Read the model definition and answer for the solid it produces. Units are mm, in the model's axes. A direction names the side the tool comes from. Coordinates: 2 decimals unless noted, no trailing zeros. Order: outer loops, then holes, each group sorted by start corner. A loop starts at its lowest first (then second) coordinate and runs counter-clockwise, first axis right, second up.
```python
from build123d import *

# Parameters (mm, degrees)
SKETCH1_W           = 37.5
SKETCH1_H           = 37.5
BOSS_EXTRUDE1_DEPTH = 15
SHELL1_T            = 2.25
CUT_EXTRUDE1_REACH  = 52.026
SKETCH2_W           = 25
SKETCH2_H           = 11
CUT_EXTRUDE2_REACH  = 52.026
SKETCH3_W           = 18
SKETCH3_H           = 9
CUT_EXTRUDE3_REACH  = 36.345
SKETCH5_W           = 29
SKETCH5_H           = 29
FILLET1_R           = 2
CUT_EXTRUDE4_REACH  = 52.026
SKETCH6_W           = 22
SKETCH6_H           = 14
FILLET2_R           = 1
SKETCH9_W           = 12
SKETCH9_H           = 10
BOSS_EXTRUDE3_DEPTH = 5
BOSS_EXTRUDE4_DEPTH = 10
SKETCH11_R          = 1.65
CUT_EXTRUDE5_DEPTH  = 5
CUT_EXTRUDE6_REACH  = 42.989
SKETCH12_R          = 3
CUT_EXTRUDE7_REACH  = 44.75
MIRROR3_OUTLINE_R   = 1.65
MIRROR3_DEPTH       = 5
MIRROR3_START       = 5
MIRROR3_2_OUTLINE_R = 3
MIRROR3_2_DEPTH     = 12.25
MIRROR3_START_2     = 27.072732359
MIRROR3_3_OUTLINE_W = 20
MIRROR3_3_OUTLINE_H = 11
MIRROR3_3_DEPTH     = 9.927267641
CHAMFER1_SIZE       = 2
FILLET3_R           = 1


with BuildPart() as part:
    # Sketch1 → Boss-Extrude1 (new body)
    with BuildSketch(Plane(origin=(0, 0, 0), x_dir=(1, 0, 0), z_dir=(0, 1, 0))):
        Rectangle(SKETCH1_W, SKETCH1_H)
    extrude(amount=BOSS_EXTRUDE1_DEPTH)

    # Shell1
    shell1_openings = [part.faces().sort_by_distance(p)[0] for p in [
        (0, 0, 0),
    ]]
    offset(amount=SHELL1_T, openings=shell1_openings, kind=Kind.INTERSECTION)

    # Sketch2 → Cut-Extrude1 (cut, up to next)
    with BuildSketch(Plane.XY.offset(21), mode=Mode.PRIVATE) as cut_extrude1_sk1:
        with Locations((0, 5.5)):
            Rectangle(SKETCH2_W, SKETCH2_H)
    cut_extrude1_tool1 = extrude(cut_extrude1_sk1.sketch, amount=-CUT_EXTRUDE1_REACH, mode=Mode.PRIVATE) & part.part
    add(cut_extrude1_tool1.solids().sort_by_distance((0, 5.5, 21))[0], mode=Mode.SUBTRACT)

    # Sketch3 → Cut-Extrude2 (cut, up to next)
    with BuildSketch(Plane(origin=(21, 0, 0), x_dir=(0, 0, -1), z_dir=(1, 0, 0)), mode=Mode.PRIVATE) as cut_extrude2_sk1:
        with Locations((-2, 4.5)):
            Rectangle(SKETCH3_W, SKETCH3_H)
    cut_extrude2_tool1 = extrude(cut_extrude2_sk1.sketch, amount=-CUT_EXTRUDE2_REACH, mode=Mode.PRIVATE) & part.part
    add(cut_extrude2_tool1.solids().sort_by_distance((21, 4.5, 2))[0], mode=Mode.SUBTRACT)

    # Sketch5 → Cut-Extrude3 (cut, up to next)
    with BuildSketch(Plane(origin=(0, 17.25, 0), x_dir=(1, 0, 0), z_dir=(0, 1, 0)), mode=Mode.PRIVATE) as cut_extrude3_sk1:
        Rectangle(SKETCH5_W, SKETCH5_H)
    cut_extrude3_tool1 = extrude(cut_extrude3_sk1.sketch, amount=-CUT_EXTRUDE3_REACH, mode=Mode.PRIVATE) & part.part
    add(cut_extrude3_tool1.solids().sort_by_distance((0, 17.25, 0))[0], mode=Mode.SUBTRACT)

    # Fillet1
    fillet1_edges = [part.edges().sort_by_distance(p)[0] for p in [
        (14.5, 16.125, -14.5),
        (14.5, 16.125, 14.5),
        (-14.5, 16.125, 14.5),
        (-14.5, 16.125, -14.5),
    ]]
    fillet(fillet1_edges, radius=FILLET1_R)

    # Sketch6 → Cut-Extrude4 (cut, up to next)
    with BuildSketch(Plane(origin=(0, 0, -21), x_dir=(-1, 0, 0), z_dir=(0, 0, -1)), mode=Mode.PRIVATE) as cut_extrude4_sk1:
        with Locations((0, 7)):
            Rectangle(SKETCH6_W, SKETCH6_H)
    cut_extrude4_tool1 = extrude(cut_extrude4_sk1.sketch, amount=-CUT_EXTRUDE4_REACH, mode=Mode.PRIVATE) & part.part
    add(cut_extrude4_tool1.solids().sort_by_distance((0, 7, -21))[0], mode=Mode.SUBTRACT)

    # Fillet2
    fillet2_edges = [part.edges().sort_by_distance(p)[0] for p in [
        (-11, 14, -19.875),
        (11, 14, -19.875),
        (12.5, 11, 19.875),
        (-12.5, 11, 19.875),
        (19.875, 9, 11),
        (19.875, 9, -7),
    ]]
    fillet(fillet2_edges, radius=FILLET2_R)

    # Sketch9 → Boss-Extrude3 (add)
    with BuildSketch(Plane.XZ):
        with Locations((-27, 16)):
            Rectangle(SKETCH9_W, SKETCH9_H)
    boss_extrude3 = extrude(amount=-BOSS_EXTRUDE3_DEPTH)

    # Sketch10 → Boss-Extrude4 (add)
    with BuildSketch(Plane.XY.offset(21)):
        Polygon((-21, 17.25), (-33, 5), (-21, 5), align=None)
    boss_extrude4 = extrude(amount=-BOSS_EXTRUDE4_DEPTH)

    # Sketch11 → Cut-Extrude5 (cut)
    with BuildSketch(Plane.XZ):
        with Locations(Location((-28, 16, 0), (0, 0, 270))):
            Circle(SKETCH11_R)
    cut_extrude5 = extrude(amount=-CUT_EXTRUDE5_DEPTH, mode=Mode.SUBTRACT)

    # Cut-Extrude6: up to this plane
    cut_extrude6_end = Plane(origin=(-21, 17.25, -6.14825064), z_dir=(-0.7143585813751187, 0.6997798348164429, 0))
    # Sketch12 → Cut-Extrude6 (cut, up to the surface)
    with BuildSketch(Plane.XZ.offset(-5), mode=Mode.PRIVATE) as cut_extrude6_sk1:
        with Locations(Location((-28, 16, 0), (0, 0, 270))):
            Circle(SKETCH12_R)
    cut_extrude6_tool1 = split(extrude(cut_extrude6_sk1.sketch, amount=-CUT_EXTRUDE6_REACH, mode=Mode.PRIVATE), bisect_by=cut_extrude6_end, keep=Keep.BOTH, mode=Mode.PRIVATE)
    cut_extrude6 = cut_extrude6_tool1.solids().sort_by_distance((-28, 5, 16))[0]
    add(cut_extrude6, mode=Mode.SUBTRACT)

    # Cut-Extrude7: up to this plane
    cut_extrude7_end = Plane(origin=(-21, 17.25, -6.14825064), z_dir=(-0.7143585813751187, 0.6997798348164429, 0))
    # Sketch13 → Cut-Extrude7 (cut, up to the surface)
    with BuildSketch(Plane.XZ, mode=Mode.PRIVATE) as cut_extrude7_sk1:
        with BuildLine():
            ThreePointArc((-33, 16), (-31.535533906, 19.535533906), (-28, 21))
            Line((-28, 21), (-33, 21))
            Line((-33, 21), (-33, 16))
        make_face()
    cut_extrude7_tool1 = split(extrude(cut_extrude7_sk1.sketch, amount=-CUT_EXTRUDE7_REACH, mode=Mode.PRIVATE), bisect_by=cut_extrude7_end, keep=Keep.BOTH, mode=Mode.PRIVATE)
    # Sketch13 → Cut-Extrude7 (cut, up to the surface)
    with BuildSketch(Plane.XZ, mode=Mode.PRIVATE) as cut_extrude7_sk2:
        with BuildLine():
            Line((-33, 11), (-28, 11))
            ThreePointArc((-28, 11), (-31.535533906, 12.464466094), (-33, 16))
            Line((-33, 16), (-33, 11))
        make_face()
    cut_extrude7_tool2 = split(extrude(cut_extrude7_sk2.sketch, amount=-CUT_EXTRUDE7_REACH, mode=Mode.PRIVATE), bisect_by=cut_extrude7_end, keep=Keep.BOTH, mode=Mode.PRIVATE)
    cut_extrude7 = cut_extrude7_tool1.solids().sort_by_distance((-31.88316, 0, 19.88316))[0] + cut_extrude7_tool2.solids().sort_by_distance((-31.88316, 0, 12.11684))[0]
    add(cut_extrude7, mode=Mode.SUBTRACT)

    # Mirror1: Boss-Extrude3, Boss-Extrude4, Cut-Extrude5, Cut-Extrude6, Cut-Extrude7 across plane
    add(boss_extrude3.mirror(Plane.XY))
    add(boss_extrude4.mirror(Plane.XY))
    add(cut_extrude5.mirror(Plane.XY), mode=Mode.SUBTRACT)
    add(cut_extrude6.mirror(Plane.XY), mode=Mode.SUBTRACT)
    add(cut_extrude7.mirror(Plane.XY), mode=Mode.SUBTRACT)

    # Mirror3: read off the stored shape, not the designer's step
    # Mirror3 outline → Mirror3 (add)
    # profile 1 of 2: a face of its own
    with BuildSketch(Plane(origin=(0, 0, 0), x_dir=(1, 0, 0), z_dir=(0, 1, 0))):
        with BuildLine():
            Line((21, 21), (21, 11))
            Line((21, 11), (28, 11))
            ThreePointArc((28, 11), (33, 16), (28, 21))
            Line((28, 21), (21, 21))
        make_face()
        with Locations((28, 16)):
            Circle(MIRROR3_OUTLINE_R, mode=Mode.SUBTRACT)
    # profile 2 of 2: a face of its own
    with BuildSketch(Plane(origin=(0, 0, 0), x_dir=(1, 0, 0), z_dir=(0, 1, 0))):
        with BuildLine():
            Line((28, -11), (21, -11))
            Line((21, -11), (21, -21))
            Line((21, -21), (28, -21))
            ThreePointArc((28, -21), (33, -16), (28, -11))
        make_face()
        with Locations((28, -16)):
            Circle(MIRROR3_OUTLINE_R, mode=Mode.SUBTRACT)
    extrude(amount=MIRROR3_DEPTH)

    # Mirror3 2 outline → Mirror3 2 (add)
    # profile 1 of 2: a face of its own
    with BuildSketch(Plane(origin=(0, 0, 0), x_dir=(1, 0, 0), z_dir=(0, 1, 0)).offset(MIRROR3_START)):
        with BuildLine():
            Line((21, 21), (21, 11))
            Line((21, 11), (28, 11))
            ThreePointArc((28, 11), (33, 16), (28, 21))
            Line((28, 21), (21, 21))
        make_face()
        with Locations((28, 16)):
            Circle(MIRROR3_2_OUTLINE_R, mode=Mode.SUBTRACT)
    # profile 2 of 2: a face of its own
    with BuildSketch(Plane(origin=(0, 0, 0), x_dir=(1, 0, 0), z_dir=(0, 1, 0)).offset(MIRROR3_START)):
        with BuildLine():
            Line((28, -11), (21, -11))
            Line((21, -11), (21, -21))
            Line((21, -21), (28, -21))
            ThreePointArc((28, -21), (33, -16), (28, -11))
        make_face()
        with Locations((28, -16)):
            Circle(MIRROR3_2_OUTLINE_R, mode=Mode.SUBTRACT)
    extrude(amount=MIRROR3_2_DEPTH)

    # Mirror3 3 outline → Mirror3 3 (cut)
    with BuildSketch(Plane(origin=(0, 0, 0), x_dir=(0.6997798348164427, -0.7143585813751188, 0), z_dir=(0.7143585813751188, 0.6997798348164428, 0)).offset(MIRROR3_START_2)):
        with Locations((11, 16.5)):
            Rectangle(MIRROR3_3_OUTLINE_W, MIRROR3_3_OUTLINE_H)
        with Locations((11, -16.5)):
            Rectangle(MIRROR3_3_OUTLINE_W, MIRROR3_3_OUTLINE_H)
    extrude(amount=MIRROR3_3_DEPTH, mode=Mode.SUBTRACT)

    # Chamfer1
    chamfer1_edges = [part.edges().sort_by_distance(p)[0] for p in [
        (-21, 8.625, 11),
        (-21, 8.625, -11),
        (21, 8.625, -11),
    ]]
    chamfer(chamfer1_edges, length=CHAMFER1_SIZE)

    # Fillet3
    fillet3_edges = [part.edges().sort_by_distance(p)[0] for p in [
        (18.75, 7.5, 18.75),
        (18.75, 7.5, -18.75),
        (-18.75, 7.5, -18.75),
        (-18.75, 7.5, 18.75),
    ]]
    fillet(fillet3_edges, radius=FILLET3_R)


solid = part.part
```
1) Straight lines are drawn through the part: line 1 (X direction, y = 3.4, z = 16); line 2 (Z direction, x = 28, y = 3); line 3 (Z direction, x = 28, y = 10). For each, find the intervals that lie inside material, in ascending order.
A:
line 1: x = -33 to -29.65, -26.35 to -18.75, 18.75 to 26.35, 29.65 to 33
line 2: z = -21 to -17.65, -14.35 to -11, 11 to 14.35, 17.65 to 21
line 3: z = -21 to -19, -13 to -11, 11 to 13, 19 to 21
2) A cutting plane is placed at A-A, the plane x = -3. Determine the outline of the cut face in (y, z).
A:
outline: (11, 18.75) - (15, 18.75) - (15, 14.5) - (17.25, 14.5) - (17.25, 21) - (11, 21) - close; (14, -21) - (17.25, -21) - (17.25, -14.5) - (15, -14.5) - (15, -18.75) - (14, -18.75) - close
3) Determine the mould class of faces 1 (the flat face through (-25.583, 12.572, -13.751)), 2 (the flat face through (-26, 6, -11)), 3 (the cylindrical face through (25, 8, -16)) for opening direction X: pulls with the +X half, pulls with the -X half, needs draft (parallel to the pull), parting line crosses it, or undercut.
A:
face 1: pulls with the -X half
face 2: needs draft
face 3: undercut
4) A cutting plane is placed at C-C, the plane y = 3.75. State how many separate pieces and enclosed holes the cut face has, and give its area (3 significant figures).
A:
separate pieces: 3
enclosed holes: 4
area: 621 mm2
5) Which of the six approach directions +Z, -Z, +X, -X, +Y, -Y give full straight-line access (tool end or side, diameter ignored) to faces 4 (the cylindrical face through (-25, 8, 16)), 5 (the flat face through (20, 9, 2)), 6 (the cylindrical face through (13.9, 16.11, 13.93)), 7 (the flat face through (-18.75, 7, 0))?
A:
face 4: +Y
face 5: +X, -Y
face 6: +Y, -Y
face 7: -Y
6) A cutting plane is placed at B-B, the plane z = 2. Determine the outline of the cut face in (x, y).
A:
outline: (-21, 0) - (-18.75, 0) - (-18.75, 15) - (-14.5, 15) - (-14.5, 17.25) - (-21, 17.25) - close; (14.5, 15) - (18.75, 15) - (18.75, 9) - (21, 9) - (21, 17.25) - (14.5, 17.25) - close
7) Flat-ended cylindrical pins translate along their axes: pin 1 Ø2.5 at (y, z) = (6, 20) entering from -X; pin 2 Ø10 at (y, z) = (4.5, 0.5) entering from -X; pin 3 Ø1.1 at (y, z) = (16, 2.5) entering from +X. Find the tip coordinate at first contact, or state that the pin passes through.
A:
pin 1: stops at x = -32.17
pin 2: stops at x = -21
pin 3: stops at x = 21
